Can you work these out from the drawing? Everything is in mm from the part's minimum corner. Give positions to 0.01 mm unless a question says otherwise; leave off trailing zeros. Loops run counter-clockwise (first coordinate to the right, second up) from the corner with the lowest first, then second, coordinate; pieces in that order, holes last. Notation, with made-up numbers: (-30.75, 4) -> (13.25, 4) arc R22 ccw to (13.25, 40) -> close; hole circle Ø5 at (17, 30.25). An arc over 180 degrees is marked (long way). Write item = value, one per line. Start each with the question number.
1) I want a section at A-A (z = 80). List the corners of the cut face in (x, y) for me, and give its area (3 significant figures).
2) I want a section at C-C (y = 6.5). Count the separate pieces of the cut face and the enclosed holes in it, and give its area (3 significant figures).
3) I need wall thicknesses on probe 1 along X at (y, z) = (6, 69.5). Which ranges of the line are inside material? Lowest first, please. Write a range as from..to.
4) I'm going to push a flat-ended pin straight in: pin 1 Ø6.5 at (x, z) = (9.525, 193.675) entering from +Y. Where does the tip first touch, or does it pass through?
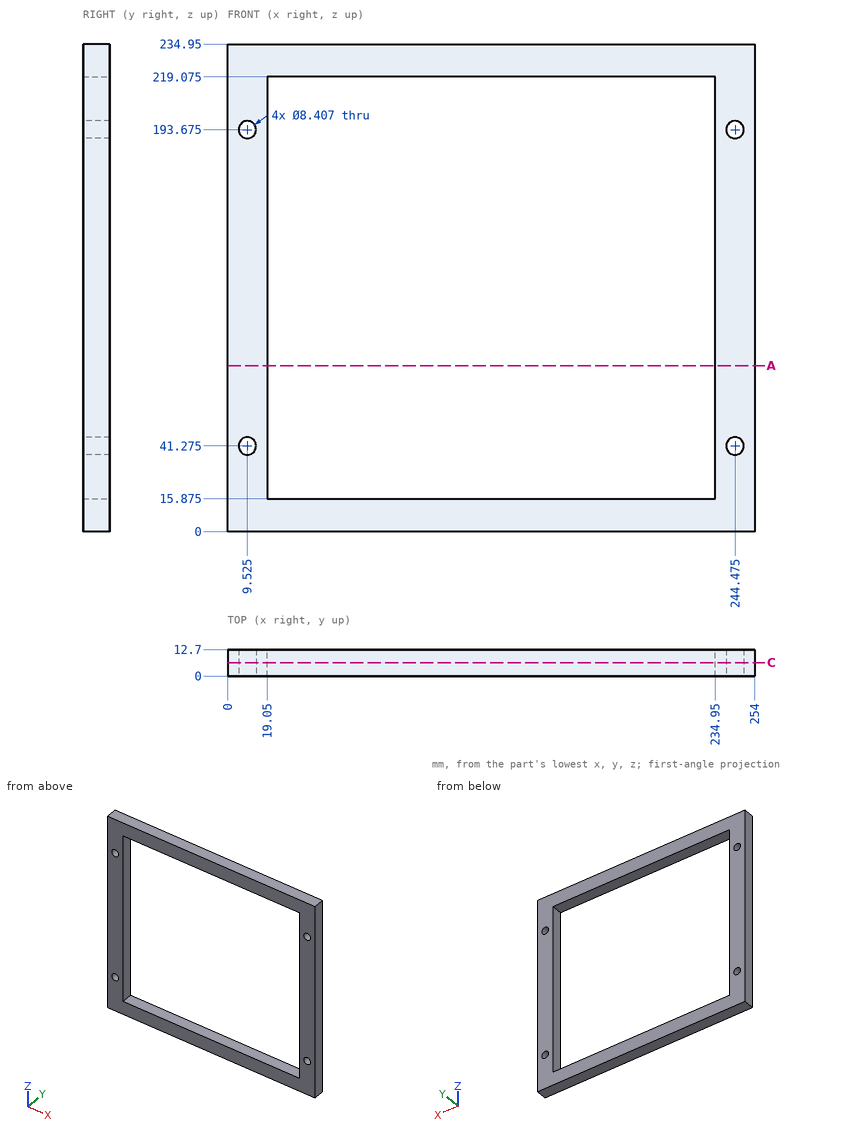
Answer list:
q1.outline = (0, 0) -> (19.05, 0) -> (19.05, 12.7) -> (0, 12.7) -> close; (234.95, 0) -> (254, 0) -> (254, 12.7) -> (234.95, 12.7) -> close
q1.area = 484 mm^2
q2.separate_pieces = 1
q2.enclosed_holes = 5
q2.area = 15,600 mm^2
q3.probe_1 = 0..19.05, 234.95..254
q4.pin_1 = through
